```python
from build123d import *

# Parameters (mm, degrees)
SKETCH_W     = 24
SKETCH_H     = 74
SKETCH_R     = 1.75
PAD_DEPTH    = 5
SKETCH001_R  = 1.75
POCKET_DEPTH = 3
FILLET_R     = 8
FILLET001_R  = 1


with BuildPart() as part:
    # Sketch → Pad (new body)
    with BuildSketch(Plane.XY):
        with Locations((0, 8)):
            Rectangle(SKETCH_W, SKETCH_H)
        Circle(SKETCH_R, mode=Mode.SUBTRACT)
        with Locations((0, -20)):
            Circle(SKETCH_R, mode=Mode.SUBTRACT)
        with BuildLine():
            ThreePointArc((-6.85, 10), (-5.25, 8.4), (-3.65, 10))
            Line((-3.65, 10), (-3.65, 30))
            ThreePointArc((-3.65, 30), (-5.25, 31.6), (-6.85, 30))
            Line((-6.85, 10), (-6.85, 30))
        make_face(mode=Mode.SUBTRACT)
        with BuildLine():
            ThreePointArc((3.65, 10), (5.25, 8.4), (6.85, 10))
            Line((6.85, 10), (6.85, 30))
            ThreePointArc((6.85, 30), (5.25, 31.6), (3.65, 30))
            Line((3.65, 10), (3.65, 30))
        make_face(mode=Mode.SUBTRACT)
    extrude(amount=PAD_DEPTH)

    # Sketch001 → Pocket (cut)
    with BuildSketch(Plane.XY):
        Circle(SKETCH001_R)
        with Locations((0, -20)):
            Circle(SKETCH001_R)
        with BuildLine():
            ThreePointArc((1.25, 10), (5.25, 6), (9.25, 10))
            Line((9.25, 10), (9.25, 30))
            ThreePointArc((9.25, 30), (5.25, 34), (1.25, 30))
            Line((1.25, 10), (1.25, 30))
        make_face()
        with BuildLine():
            ThreePointArc((-9.25, 10), (-5.25, 6), (-1.25, 10))
            Line((-1.25, 10), (-1.25, 30))
            ThreePointArc((-1.25, 30), (-5.25, 34), (-9.25, 30))
            Line((-9.25, 10), (-9.25, 30))
        make_face()
    extrude(amount=POCKET_DEPTH, mode=Mode.SUBTRACT)

    # Fillet
    fillet_edges = [part.edges().sort_by_distance(p)[0] for p in [
        (-12, -29, 2.5),
        (12, -29, 2.5),
        (12, 45, 2.5),
        (-12, 45, 2.5),
    ]]
    fillet(fillet_edges, radius=FILLET_R)

    # Fillet001
    fillet001_edges = [part.edges().sort_by_distance(p)[0] for p in [
        (-12, 8, 0),
        (-9.656854, -26.656854, 0),
        (0, -29, 0),
        (9.656854, -26.656854, 0),
        (12, 8, 0),
        (0, 45, 0),
        (-9.656854, 42.656854, 0),
        (9.656854, 42.656854, 0),
    ]]
    fillet(fillet001_edges, radius=FILLET001_R)


solid = part.part
```
For this review, take the finished solid that the model builds, in its own axes (mm). A direction names the side the tool comes from. Coordinates: 2 decimals unless noted, no trailing zeros. Order: outer loops, then holes, each group sorted by start corner. A loop starts at its lowest first (then second) coordinate and runs counter-clockwise, first axis right, second up. Notation, with made-up numbers: (37.5, 40) -> (74.5, 40) arc R16 ccw to (74.5, 48) -> close; hole circle Ø4 at (-13, -37). An arc over 180 degrees is marked (long way). Use CSV: the item, a comma, the result in double quotes. Start each with the question number.
Item 1: Draft analysis for pull direction Y (two halves, no side actions). For faces 1 (the face through (-0.228, -18.265, 2.465)), 2 (the face through (-6.85, 20, 4)), 3 (the face through (12, 8, 3)), 4 (the face through (-9.719, 42.594, 3.028)), state which applies: pulls with the +Y half, pulls with the -Y half, needs draft (parallel to the pull), parting line crosses it, or undercut.
Item 2: We need section B-B, the plane x = 0. Give the boundary of the cut face in (y, z).
Item 3: We need section C-C, the plane y = 28. Give the boundary of the cut face in (x, z).
Item 4: Wall thickness on probe 1 along Y at (x, z) = (0, 1.55); probe 2 along X at (y, z) = (10, 4.05); probe 3 along Y at (x, z) = (-1.5, 4.8): over which ranges is each line inside the solid? List them lowest first.
Item 5: We need section A-A, the plane y = -20. Give the boundary of the cut face in (x, z).
Item 6: For faces 5 (the face through (-9.25, 20, 1)), 6 (the face through (3.65, 20, 4)), 7 (the face through (-12, 8, 3)), list the 3-axis set-ups (+Z, -Z, +X, -X, +Y, -Y) from which the entire face can be reached by the end or side of a thin tool; tool diameter is ignored.
Derived:
1,face 1,"undercut"
1,face 2,"undercut"
1,face 3,"needs draft"
1,face 4,"pulls with the +Y half"
2,outline,"(-29, 1) arc R1 ccw to (-28, 0) -> (-21.75, 0) -> (-21.75, 5) -> (-29, 5) -> close; (-18.25, 0) -> (-1.75, 0) -> (-1.75, 5) -> (-18.25, 5) -> close; (1.75, 0) -> (44, 0) arc R1 ccw to (45, 1) -> (45, 5) -> (1.75, 5) -> close"
3,outline,"(-12, 1) arc R1 ccw to (-11, 0) -> (-9.25, 0) -> (-9.25, 3) -> (-6.85, 3) -> (-6.85, 5) -> (-12, 5) -> close; (-3.65, 3) -> (-1.25, 3) -> (-1.25, 0) -> (1.25, 0) -> (1.25, 3) -> (3.65, 3) -> (3.65, 5) -> (-3.65, 5) -> close; (6.85, 3) -> (9.25, 3) -> (9.25, 0) -> (11, 0) arc R1 ccw to (12, 1) -> (12, 5) -> (6.85, 5) -> close"
4,probe 1,"y = -29 to -21.75, -18.25 to -1.75, 1.75 to 45"
4,probe 2,"x = -12 to -6.85, -3.65 to 3.65, 6.85 to 12"
4,probe 3,"y = -29 to -20.9, -19.1 to -0.9, 0.9 to 45"
5,outline,"(-12, 1) arc R1 ccw to (-11, 0) -> (-1.75, 0) -> (-1.75, 5) -> (-12, 5) -> close; (1.75, 0) -> (11, 0) arc R1 ccw to (12, 1) -> (12, 5) -> (1.75, 5) -> close"
6,face 5,"-Z"
6,face 6,"+Z, -Z"
6,face 7,"+Z, -Z, -X, +Y, -Y"
